from build123d import *

# Parameters (mm, degrees)
SALIENTE_EXTRUIR1_DEPTH = 1.6
CROQUIS2_R              = 3.45
SALIENTE_EXTRUIR2_DEPTH = 1.4
CORTAR_EXTRUIR1_REACH   = 5
CROQUIS3_R              = 1.25


with BuildPart() as part:
    # Croquis1 → Saliente-Extruir1 (new body)
    with BuildSketch(Plane(origin=(0, 0, 0), x_dir=(1, 0, 0), z_dir=(0, 1, 0))):
        with BuildLine():
            Line((1, 0), (14, 0))
            ThreePointArc((14, 0), (14.707106781, 0.292893219), (15, 1))
            Line((15, 1), (15, 9))
            ThreePointArc((15, 9), (14.707106781, 9.707106781), (14, 10))
            Line((14, 10), (1, 10))
            ThreePointArc((1, 10), (0.292893219, 9.707106781), (0, 9))
            Line((0, 9), (0, 1))
            ThreePointArc((0, 1), (0.292893219, 0.292893219), (1, 0))
        make_face()
    extrude(amount=SALIENTE_EXTRUIR1_DEPTH)

    # Croquis2 → Saliente-Extruir2 (add)
    with BuildSketch(Plane(origin=(0, 1.6, 0), x_dir=(1, 0, 0), z_dir=(0, 1, 0))):
        with Locations((7.5, 5)):
            Circle(CROQUIS2_R)
    extrude(amount=SALIENTE_EXTRUIR2_DEPTH)

    # Croquis3 → Cortar-Extruir1 (cut, up to next)
    with BuildSketch(Plane(origin=(0, 3, 0), x_dir=(1, 0, 0), z_dir=(0, 1, 0)), mode=Mode.PRIVATE) as cortar_extruir1_sk1:
        with Locations((7.5, 5)):
            Circle(CROQUIS3_R)
    cortar_extruir1_tool1 = extrude(cortar_extruir1_sk1.sketch, amount=-CORTAR_EXTRUIR1_REACH, mode=Mode.PRIVATE) & part.part
    add(cortar_extruir1_tool1.solids().sort_by_distance((7.5, 3, -5))[0], mode=Mode.SUBTRACT)


solid = part.part
Design review of the part built by this model. Coordinates are the model's own, in mm. A direction names the side the tool comes from. Coordinates: 2 decimals unless noted, no trailing zeros. Loops run counter-clockwise (first coordinate to the right, second up) from the corner with the lowest first, then second, coordinate; pieces in that order, holes last.
Item 1: For faces 1 (the flat face through (4, 1.6, -6)), 2 (the flat face through (6, 0, -5)), list the 3-axis set-ups (+Z, -Z, +X, -X, +Y, -Y) from which the entire face can be reached by the end or side of a thin tool; tool diameter is ignored.
Completed:
face 1: +Y
face 2: +Z, -Z, +X, -X, -Y
Item 2: Add section B-B (y = 0.9). Write out the cut boundary in (x, z).
Completed:
outline: (0, -9) arc R1 ccw to (1, -10) - (14, -10) arc R1 ccw to (15, -9) - (15, -1) arc R1 ccw to (14, 0) - (1, 0) arc R1 ccw to (0, -1) - close; hole circle Ø2.5 at (7.5, -5)
Item 3: Add section D-D (x = 10.75). Write out the cut boundary in (y, z), and give its area (3 significant figures).
Completed:
outline: (0, -10) - (1.6, -10) - (1.6, -6.16) - (3, -6.16) - (3, -3.84) - (1.6, -3.84) - (1.6, 0) - (0, 0) - close
area: 19.2 mm2
Item 4: Add section A-A (x = 7.5). Write out the cut boundary in (y, z).
Completed:
outline: (0, -10) - (1.6, -10) - (1.6, -8.45) - (3, -8.45) - (3, -6.25) - (0, -6.25) - close; (0, -3.75) - (3, -3.75) - (3, -1.55) - (1.6, -1.55) - (1.6, 0) - (0, 0) - close
Item 5: Wall thickness on L1, parallel to X at y = 1.4, z = -5; L2, parallel to Z at x = 7.5, y = 1.1; L3, parallel to Z at x = 7.5, y = 1.65: over which ranges is each line inside the solid? List them lowest first.
Completed:
L1: x = 0 to 6.25, 8.75 to 15
L2: z = -10 to -6.25, -3.75 to 0
L3: z = -8.45 to -6.25, -3.75 to -1.55
Item 6: Clearance check with a flat-ended pin moving along its axis: pin 1 (4 mm diameter, centred on x = 7.5, z = -5, fed in from -Y). State where the tip first meets the part, or that it passes through.
Completed:
pin 1: stops at y = 0
Item 7: Draft analysis for pull direction Z (two halves, no side actions). For faces 3 (the cylindrical face through (6.51, 1.52, -4.24)), 4 (the cylindrical face through (14.699, 0.789, -0.285)), 5 (the cylindrical face through (10.8, 2.3, -6)), 6 (the cylindrical face through (14.715, 0.789, -9.699)), state which applies: pulls with the +Z half, pulls with the -Z half, needs draft (parallel to the pull), parting line crosses it, or undercut.
Completed:
face 3: undercut
face 4: pulls with the +Z half
face 5: parting line crosses it
face 6: pulls with the -Z half
Item 8: Add section C-C (z = -4.5). Write out the cut boundary in (x, y), and give its area (3 significant figures).
Completed:
outline: (0, 0) - (6.35, 0) - (6.35, 3) - (4.09, 3) - (4.09, 1.6) - (0, 1.6) - close; (8.65, 0) - (15, 0) - (15, 1.6) - (10.91, 1.6) - (10.91, 3) - (8.65, 3) - close
area: 26.7 mm2
